```python
from build123d import *

# Parameters (mm, degrees)
SKETCH_1_W               = 40
SKETCH_1_H               = 30
EXTRUDE_1_DEPTH          = 5
SKETCH_2_W               = 25.5
SKETCH_2_H               = 30
EXTRUDE_2_DEPTH          = 5
SKETCH_3_W               = 5
SKETCH_3_H               = 30
EXTRUDE_3_DEPTH          = 30.5
SKETCH_5_W               = 30.5
SKETCH_5_H               = 30
EXTRUDE_4_DEPTH          = 5
SKETCH_6_W               = 5
SKETCH_6_H               = 30
EXTRUDE_5_DEPTH          = 40
RIB_1_REACH              = 106.645
SKETCH_9_WALL_W          = 238.652565268
SKETCH_9_WALL_H          = 10
MIRROR_2_COPY_1_REACH    = 106.645
MIRROR_2_COPY_1_SKETCH_W = 238.652565268
MIRROR_2_COPY_1_SKETCH_H = 10
SKETCH_10_R              = 1.75
CUT_EXTRUDE_1_DEPTH      = 82
SKETCH_11_R              = 1.75
CUT_EXTRUDE_2_DEPTH      = 40
SKETCH_12_W              = 35.5
SKETCH_12_H              = 30
EXTRUDE_6_DEPTH          = 5
SKETCH_13_R              = 1.75
CUT_EXTRUDE_3_DEPTH      = 66


with BuildPart() as part:
    # 草图1 → 凸台-拉伸1 (new body)
    with BuildSketch(Plane.XY):
        Rectangle(SKETCH_1_W, SKETCH_1_H)
    extrude(amount=EXTRUDE_1_DEPTH)

    # 草图2 → 凸台-拉伸2 (add)
    with BuildSketch(Plane(origin=(20, 0, 0), x_dir=(0, 0, -1), z_dir=(1, 0, 0))):
        with Locations((-12.75, 0)):
            Rectangle(SKETCH_2_W, SKETCH_2_H)
    extrude(amount=EXTRUDE_2_DEPTH)

    # 草图3 → 凸台-拉伸3 (add)
    with BuildSketch(Plane.ZY.offset(-20)):
        with Locations((28, 0)):
            Rectangle(SKETCH_3_W, SKETCH_3_H)
    extrude(amount=-EXTRUDE_3_DEPTH)

    # 草图5 → 凸台-拉伸4 (add)
    with BuildSketch(Plane(origin=(50.5, 0, 0), x_dir=(0, 0, -1), z_dir=(1, 0, 0))):
        with Locations((-15.25, 0)):
            Rectangle(SKETCH_5_W, SKETCH_5_H)
    extrude(amount=EXTRUDE_4_DEPTH)

    # 草图6 → 凸台-拉伸5 (add)
    with BuildSketch(Plane(origin=(55.5, 0, 0), x_dir=(0, 0, -1), z_dir=(1, 0, 0))):
        with Locations((-2.5, 0)):
            Rectangle(SKETCH_6_W, SKETCH_6_H)
    extrude(amount=EXTRUDE_5_DEPTH)

    # 草图9 wall → 筋1 (add, up to next)
    with BuildSketch(Plane(origin=(65.5, -15, 14.337421174), x_dir=(0.730906214245, 0, -0.68247791611), z_dir=(0.68247791611, 0, 0.730906214245)), mode=Mode.PRIVATE) as rib_1_sk1:
        with Locations((0, 5)):
            Rectangle(SKETCH_9_WALL_W, SKETCH_9_WALL_H)
    rib_1_tool1 = extrude(rib_1_sk1.sketch, amount=-RIB_1_REACH, mode=Mode.PRIVATE) - part.part
    rib_1 = rib_1_tool1.solids().sort_by_distance((65.5, -15, 14.337421174))[0]
    add(rib_1)

    # 镜向1: 筋1 across plane
    add(rib_1.mirror(Plane.ZX))

    # 镜向2: 筋1 across plane
    add(rib_1.mirror(Plane(origin=(37.75, 0, 0), x_dir=(0, 0, 1), z_dir=(1, 0, 0))))

    # 镜向2 copy 1 sketch → 镜向2 copy 1 (add, up to next)
    with BuildSketch(Plane(origin=(10, 15, 14.337421174), x_dir=(-0.730906214245, 0, -0.68247791611), z_dir=(-0.68247791611, 0, 0.730906214245)), mode=Mode.PRIVATE) as mirror_2_copy_1_sk1:
        with Locations((0, 5)):
            Rectangle(MIRROR_2_COPY_1_SKETCH_W, MIRROR_2_COPY_1_SKETCH_H)
    mirror_2_copy_1_tool1 = extrude(mirror_2_copy_1_sk1.sketch, amount=-MIRROR_2_COPY_1_REACH, mode=Mode.PRIVATE) - part.part
    add(mirror_2_copy_1_tool1.solids().sort_by_distance((10, 15, 14.337421174))[0])

    # 草图10 → 切除-拉伸1 (cut)
    with BuildSketch(Plane(origin=(0, 0, 0), x_dir=(-1, 0, 0), z_dir=(0, 0, -1))):
        with Locations((-52.75, 0)):
            Circle(SKETCH_10_R)
        with Locations((-22.75, 0)):
            Circle(SKETCH_10_R)
        with Locations((-82.75, 0)):
            Circle(SKETCH_10_R)
        with Locations((7.25, 0)):
            Circle(SKETCH_10_R)
    extrude(amount=-CUT_EXTRUDE_1_DEPTH, mode=Mode.SUBTRACT)

    # 草图11 → 切除-拉伸2 (cut)
    with BuildSketch(Plane(origin=(0, 0, 0), x_dir=(-1, 0, 0), z_dir=(0, 0, -1))):
        with Locations((-67.75, 0)):
            Circle(SKETCH_11_R)
        with Locations(Location((-7.75, 0, 0), (0, 0, 180))):
            Circle(SKETCH_11_R)
    extrude(amount=-CUT_EXTRUDE_2_DEPTH, mode=Mode.SUBTRACT)

    # 草图12 → 凸台-拉伸6 (add)
    with BuildSketch(Plane.XY.offset(30.5)):
        with Locations((37.75, 0)):
            Rectangle(SKETCH_12_W, SKETCH_12_H)
    extrude(amount=EXTRUDE_6_DEPTH)

    # 草图13 → 切除-拉伸3 (cut)
    with BuildSketch(Plane(origin=(0, 0, 0), x_dir=(-1, 0, 0), z_dir=(0, 0, -1))):
        with Locations((-22.75, 0)):
            Circle(SKETCH_13_R)
        with Locations((-52.75, 0)):
            Circle(SKETCH_13_R)
    extrude(amount=-CUT_EXTRUDE_3_DEPTH, mode=Mode.SUBTRACT)


solid = part.part
```
Geometry: final body of the model. Coordinates: model frame, mm. A direction names the side the tool comes from. Round coordinates to 2 decimals unless told otherwise and drop trailing zeros. Write each loop counter-clockwise with the first axis right and the second up, starting at its lowest first coordinate (ties: lowest second). Pieces come first, ordered by that corner, then holes. Notation, with made-up numbers: M 17,33.25 L 50,33.25 A19 cw 50,50.25 Z; hole C -20.75,-24 d2. An arc over 180 degrees is marked long. Answer in a Markdown table with one row per item. Add a question column.
(1) Cut plane A-A, the plane z = 20. Return the cut outline in (x, y).
(2) Cut plane D-D, the plane z = 33.5. Return the cut outline in (x, y), then the cut area to 3 significant figures.
(3) Draft query along X for faces 1 (the face through (24.6, 15, 12.4)), 2 (the face through (9.419, -0.526, 2.465)), 3 (the face through (95.5, 0, 3)). Return one class per face: pulls with the +X half, pulls with the -X half, needs draft (parallel to the pull), parting line crosses it, or undercut.
(4) Contact query for flat-ended pins moving along their axis: pin 1 (3 mm diameter, centred on x = 67.75, y = 0, fed in from +Z); pin 2 (1.5 mm diameter, centred on y = 4.5, z = 25.5, fed in from -X); pin 3 (15 mm diameter, centred on y = 4.5, z = 21, fed in from +X); pin 4 (5 mm diameter, centred on y = -5.5, z = 29.5, fed in from +X). Output: stop coordinate, or through.
(5) Ray query, L1, parallel to Y at x = 7.75, z = 2.1; L2, parallel to X at y = -0.75, z = 15; L3, parallel to X at y = 4, z = 13. Return the intervals inside material, ascending.
(6) Cut plane B-B, the plane x = -7.25. Return the cut outline in (y, z).
(7) Cut plane C-C, the plane y = -6.75. Return the cut outline in (x, z), then the cut area to 3 significant figures.
(8) Reachability of faces 4 (the face through (81.081, 0.526, 2.465)), 5 (the face through (55.5, 0, 23)), 6 (the face through (50.5, 0, 13)), 7 (the face through (73, 0, 0)), 8 (the face through (14, 5, 11)) from +Z, -Z, +X, -X, +Y, -Y: full face, straight path, thin tool, end or side. Return the list, or none.
Established:
| question | item | result |
|---|---|---|
| 1 | outline | M 16.06,-15 L 25,-15 L 25,15 L 16.06,15 L 16.06,5 L 20,5 L 20,-5 L 16.06,-5 Z; M 50.5,-15 L 59.44,-15 L 59.44,-5 L 55.5,-5 L 55.5,5 L 59.44,5 L 59.44,15 L 50.5,15 Z; hole C 22.75,0 d3.5; hole C 52.75,0 d3.5 |
| 2 | outline | M 20,-15 L 55.5,-15 L 55.5,15 L 20,15 Z; hole C 22.75,0 d3.5; hole C 52.75,0 d3.5 |
| 2 | area | 1,050 mm² |
| 3 | face 1 | needs draft |
| 3 | face 2 | undercut |
| 3 | face 3 | pulls with the +X half |
| 4 | pin 1 | through |
| 4 | pin 2 | x = 20 |
| 4 | pin 3 | x = 66.38 |
| 4 | pin 4 | x = 55.5 |
| 5 | L1 | -15 to -1.75, 1.75 to 15 |
| 5 | L2 | 20 to 21.17, 24.33 to 25, 50.5 to 51.17, 54.33 to 55.5 |
| 5 | L3 | 20 to 25, 50.5 to 55.5 |
| 6 | outline | M -15,0 L -1.75,0 L -1.75,5 L -15,5 Z; M 1.75,0 L 15,0 L 15,5 L 1.75,5 Z |
| 7 | outline | M -20,0 L 25,0 L 25,25.5 L 50.5,25.5 L 50.5,0 L 95.5,0 L 95.5,5 L 75.5,5 L 55.5,23.67 L 55.5,35.5 L 20,35.5 L 20,23.67 L 0,5 L -20,5 Z |
| 7 | area | 1,380 mm² |
| 8 | face 4 | +Z, -Z |
| 8 | face 5 | +Z, +X |
| 8 | face 6 | -Z, +Y, -Y |
| 8 | face 7 | -Z, +X, -X, +Y, -Y |
| 8 | face 8 | +Z, -X |
